For this review, use the dimensioned drawing (mm, ordinates from the lowest corner) and the shaded views. A direction names the side the tool comes from. Coordinates: 2 decimals unless noted, no trailing zeros. Write each loop counter-clockwise with the first axis right and the second up, starting at its lowest first coordinate (ties: lowest second). Pieces come first, ordered by that corner, then holes. Notation, with made-up numbers: (-6.75, -38) -> (49.25, -38) arc R27 cw to (49.25, -14) -> close; hole circle Ø7 at (8.25, 83). An arc over 180 degrees is marked (long way). Put each result on its own line as item: value. Start each with the question number.
Item 1: For the marked faces 1, 2 and 3, list the 3-axis set-ups (+Z, -Z, +X, -X, +Y, -Y) from which the entire face can be reached by the end or side of a thin tool; tool diameter is ignored.
Item 2: Consider section A-A on z = 25. Give the boundary of the cut face in (x, y).
Item 3: Consider section D-D on y = 5. Give the boundary of the cut face in (x, z).
Item 4: To check wall thickness, follow L1, parallel to X at y = 3.1, z = 25; L2, parallel to Z at x = 28, y = 7.25; L3, parallel to Y at x = 37, z = 10.5. State the ranges of each line that lie inside material, in increasing order.
Item 5: Consider section C-C on y = 1. Give the boundary of the cut face in (x, z), and give its area (3 significant figures).
Item 6: Insertion check: P1, Ø5, axis at y = 4.5, z = 30, coming from the +X side; P2, Ø1.5, axis at x = 9.5, y = 1.5, coming from the +Z side; P3, Ø4, axis at y = 6, z = 43.5, coming from the -X side; P4, Ø4.5, axis at x = 25, z = 25, coming from the -Y side. Each pin has a flat end and moves straight along its axis. Give the tip position at first contact, or say it passes through.
Item 7: The part is to be moulded in two halves that separate along X. For the marked faces 4, 5, 6 and 7, say which applies: +X half, -X half, draft (parallel to the pull), parting line (faces both ways), or undercut.
Item 8: Consider section B-B on x = 25. Give the boundary of the cut face in (y, z).
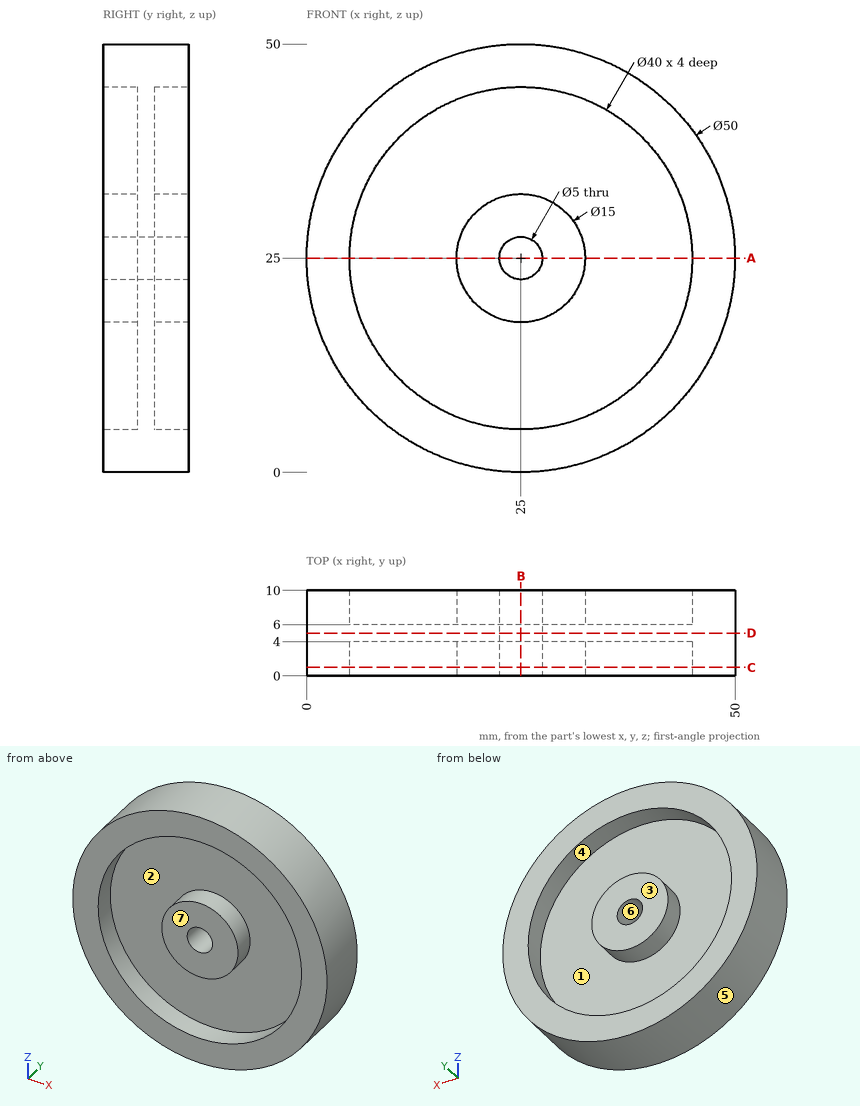
Return value:
1. face 1: +Y
1. face 2: -Y
1. face 3: +Z, -Z, +X, -X, +Y
2. outline: (0, 0) -> (5, 0) -> (5, 4) -> (17.5, 4) -> (17.5, 0) -> (22.5, 0) -> (22.5, 10) -> (17.5, 10) -> (17.5, 6) -> (5, 6) -> (5, 10) -> (0, 10) -> close; (27.5, 0) -> (32.5, 0) -> (32.5, 4) -> (45, 4) -> (45, 0) -> (50, 0) -> (50, 10) -> (45, 10) -> (45, 6) -> (32.5, 6) -> (32.5, 10) -> (27.5, 10) -> close
3. outline: circle Ø50 at (25, 25); hole circle Ø5 at (25, 25)
4. L1: 0 to 5, 17.5 to 22.5, 27.5 to 32.5, 45 to 50
4. L2: 0.18 to 5.23, 18.13 to 31.87, 44.77 to 49.82
4. L3: 4 to 6
5. outline: circle Ø50 at (25, 25); circle Ø15 at (25, 25); hole circle Ø40 at (25, 25); hole circle Ø5 at (25, 25)
5. area: 864 mm^2
6. P1: x = 49.87
6. P2: z = 45.19
6. P3: x = 6.22
6. P4: through
7. face 4: undercut
7. face 5: parting line
7. face 6: undercut
7. face 7: draft
8. outline: (0, 0) -> (10, 0) -> (10, 5) -> (6, 5) -> (6, 17.5) -> (10, 17.5) -> (10, 22.5) -> (0, 22.5) -> (0, 17.5) -> (4, 17.5) -> (4, 5) -> (0, 5) -> close; (0, 27.5) -> (10, 27.5) -> (10, 32.5) -> (6, 32.5) -> (6, 45) -> (10, 45) -> (10, 50) -> (0, 50) -> (0, 45) -> (4, 45) -> (4, 32.5) -> (0, 32.5) -> close
